from build123d import *

# Parameters (mm, degrees)
BOX002_W       = 6
BOX002_H       = 6
BOX002_DEPTH   = 10
BOX_W          = 45
BOX_H          = 159
BOX_DEPTH      = 3
CYLINDER_R     = 3
CYLINDER_DEPTH = 10
BOX001_W       = 62
BOX001_H       = 167
BOX001_DEPTH   = 2


with BuildPart() as cube002:
    # Box002 → Box002 (new body)
    with BuildSketch(Plane(origin=(55, 137, 0), x_dir=(1, 0, 0), z_dir=(0, 0, 1))):
        with Locations((3, 3)):
            Rectangle(BOX002_W, BOX002_H)
    extrude(amount=BOX002_DEPTH)


with BuildPart() as cube:
    # Box → Box (new body)
    with BuildSketch(Plane.XY):
        with Locations((22.5, 79.5)):
            Rectangle(BOX_W, BOX_H)
    extrude(amount=BOX_DEPTH)


with BuildPart() as fusion:
    # Cylinder → Cylinder (new body)
    with BuildSketch(Plane(origin=(55, 140, 0), x_dir=(1, 0, 0), z_dir=(0, 0, 1))):
        Circle(CYLINDER_R)
    extrude(amount=CYLINDER_DEPTH)

    # Fusion: union Cube
    add(cube.part)


with BuildPart() as cut001:
    # Box001 → Box001 (new body)
    with BuildSketch(Plane(origin=(-4, -4, 0), x_dir=(1, 0, 0), z_dir=(0, 0, 1))):
        with Locations((31, 83.5)):
            Rectangle(BOX001_W, BOX001_H)
    extrude(amount=BOX001_DEPTH)

    # Cut: cut Fusion
    add(fusion.part, mode=Mode.SUBTRACT)

    # Cut001: cut Cube002
    add(cube002.part, mode=Mode.SUBTRACT)


solid = cut001.part
Geometry: final body of the model. Coordinates: model frame, mm. Coordinates: 2 decimals unless noted, no trailing zeros. Order: outer loops, then holes, each group sorted by start corner. A loop starts at its lowest first (then second) coordinate and runs counter-clockwise, first axis right, second up. Notation, with made-up numbers: M 85.5,-4.5 L 141.5,-4.5 A17 cw 141.5,6.5 Z; hole C 33,55 d11. An arc over 180 degrees is marked long. One line per question, with ' | ' between items. Start each with the question number.
Item 1: Cut plane C-C, the plane z = 0.4. Return the cut outline in (x, y), then the cut area to 3 significant figures.
Item 2: Cut plane B-B, the plane x = 31. Return the cut outline in (y, z).
Item 3: Cut plane A-A, the plane y = 108.5. Return the cut outline in (x, z).
Item 4: Ray query, probe 1 along Y at (x, z) = (15, 0.85); probe 2 along X at (y, z) = (148.5, 0.4); probe 3 along Y at (x, z) = (53.5, 1.2). Return the intervals inside material, ascending. Write a range as [from, to].
Item 5: Draft query along Y for faces 1 (the flat face through (45.2, 73.7, 2)), 2 (the cylindrical face through (52, 140, 1)). Return one class per face: released by +Y, released by -Y, zero draft, split by the parting line, or undercut.
A:
1) outline: M -4,-4 L 58,-4 L 58,137 L 55,137 A3 cw 55,143 L 58,143 L 58,163 L -4,163 Z; hole M 0,0 L 45,0 L 45,159 L 0,159 Z | area: 3,170 mm2
2) outline: M -4,0 L 0,0 L 0,2 L -4,2 Z; M 159,0 L 163,0 L 163,2 L 159,2 Z
3) outline: M -4,0 L 0,0 L 0,2 L -4,2 Z; M 45,0 L 58,0 L 58,2 L 45,2 Z
4) probe 1: y = [-4, 0], [159, 163] | probe 2: x = [-4, 0], [45, 58] | probe 3: y = [-4, 137.4], [142.6, 163]
5) face 1: zero draft | face 2: undercut
